Autodesk Inventor part; units mm, degrees
ref_plane "YZ Plane" through (0, 0, 0) normal (1, 0, 0) x (0, 1, 0)
ref_plane "XZ Plane" through (0, 0, 0) normal (0, 1, 0) x (-1, 0, 0)
ref_plane "XY Plane" through (0, 0, 0) normal (0, 0, 1) x (1, 0, 0)
sketch "Sketch1" plane through (0, 0, 0) normal (0, 1, 0) x (-1, 0, 0)
  line L0 (-20, 35) -> (20, 35)
  line L1 (20, 35) -> (20, -35)
  line L2 (20, -35) -> (-20, -35)
  line L3 (-20, -35) -> (-20, 35)
  line L4 (-20, 35) -> (20, -35) construction
  line L5 (20, 35) -> (-20, -35) construction
  circle A0 centre (0, 20) radius 2
  circle A1 centre (0, -20) radius 2
  line L6 (-12.5, 25) -> (12.5, 25) construction
  line L7 (12.5, 25) -> (12.5, -25) construction
  line L8 (12.5, -25) -> (-12.5, -25) construction
  line L9 (-12.5, -25) -> (-12.5, 25) construction
  line L10 (-12.5, 25) -> (12.5, -25) construction
  line L11 (12.5, 25) -> (-12.5, -25) construction
  circle A2 centre (12.5, -25) radius 5 construction
  circle A3 centre (12.5, -25) radius 1.5
  circle A4 centre (12.5, 25) radius 1.5
  circle A5 centre (-12.5, 25) radius 1.5
  circle A6 centre (-12.5, -25) radius 1.5
  point P0 (0, 0)
  dimension "d0" = 4
  dimension "d1" = 4
  dimension "d2" = 40
  dimension "d3" = 20
  dimension "d4" = 70
  dimension "d5" = 40
  dimension "d6" = 25
  dimension "d7" = 50
  dimension "d8" = 10
  dimension "d9" = 3
  dimension "d10" = 3
  dimension "d11" = 3
  dimension "d12" = 3
extrude "Extrusion1" add sketch "Sketch1" along normal blind 5
fillet "Fillet1" radius 2 4 edges at (20, 2.5, 35) (20, 2.5, -35) (-20, 2.5, -35) (-20, 2.5, 35)
chamfer "Chamfer1" distance 1.5 angle 45 4 edges at (-11, 5, 25) (14, 5, 25) (-11, 5, -25) (14, 5, -25)
properties part number "Encoder base"
Here's how the part is built. I have some questions about the finished solid (model axes, mm). Coordinates: 2 decimals unless noted, no trailing zeros. Order: outer loops, then holes, each group sorted by start corner. A loop starts at its lowest first (then second) coordinate and runs counter-clockwise, first axis right, second up. Notation, with made-up numbers: (48, 12.5) -> (79, 12.5) arc R28 cw to (79, 30.5) -> close; hole circle Ø6 at (48.25, -36). An arc over 180 degrees is marked (long way). Return JSON: item names as keys, results as strings.
1) If we section it at B-B on z = -20: List the corners of the cut face in (x, y) for me.
Conclusion:
{"outline": "(-20, 0) -> (-2, 0) -> (-2, 5) -> (-20, 5) -> close; (2, 0) -> (20, 0) -> (20, 5) -> (2, 5) -> close"}
2) If we section it at A-A on x = 0: List the corners of the cut face in (y, z) for me, plus the area to 3 significant figures.
Conclusion:
{"outline": "(0, -35) -> (5, -35) -> (5, -22) -> (0, -22) -> close; (0, -18) -> (5, -18) -> (5, 18) -> (0, 18) -> close; (0, 22) -> (5, 22) -> (5, 35) -> (0, 35) -> close", "area": "310 mm²"}
3) If we section it at D-D on x = 12.5: List the corners of the cut face in (y, z) for me.
Conclusion:
{"outline": "(0, -35) -> (5, -35) -> (5, -28) -> (3.5, -26.5) -> (0, -26.5) -> close; (0, -23.5) -> (3.5, -23.5) -> (5, -22) -> (5, 22) -> (3.5, 23.5) -> (0, 23.5) -> close; (0, 26.5) -> (3.5, 26.5) -> (5, 28) -> (5, 35) -> (0, 35) -> close"}
4) I'm going to push a flat-ended pin straight in: P1, Ø1.8, axis at x = 12.5, z = -25, coming from the +Y side. Where does the tip first touch, or does it pass through?
Conclusion:
{"P1": "passes through"}
5) Thinking about a two-plate mould opening in X: for faces 1 (the cylindrical face through (19.43, 2.54, -34.4)), 2 (the cylindrical face through (-12.305, 1.726, -26.487)), 3 (the cylindrical face through (-19.43, 2.54, 34.4)), which applies, +X half, -X half, draft (parallel to the pull), parting line (faces both ways), or undercut?
Conclusion:
{"face 1": "+X half", "face 2": "undercut", "face 3": "-X half"}
6) If I drill on probe 1 along Z at (x, y) = (-12.5, 2.7); probe 2 along X at (y, z) = (2.35, 26); probe 3 along Z at (x, y) = (1.5, 4.8), over which ranges is the centre line in solid material (lowest first)?
Conclusion:
{"probe 1": "z = -35 to -26.5, -23.5 to 23.5, 26.5 to 35", "probe 2": "x = -20 to -13.62, -11.38 to 11.38, 13.62 to 20", "probe 3": "z = -35 to -21.32, -18.68 to 18.68, 21.32 to 35"}
7) If we section it at C-C on y = 2.55: List the corners of the cut face in (x, z) for me, plus the area to 3 significant figures.
Conclusion:
{"outline": "(-20, -33) arc R2 ccw to (-18, -35) -> (18, -35) arc R2 ccw to (20, -33) -> (20, 33) arc R2 ccw to (18, 35) -> (-18, 35) arc R2 ccw to (-20, 33) -> close; hole circle Ø3 at (-12.5, -25); hole circle Ø3 at (-12.5, 25); hole circle Ø4 at (0, -20); hole circle Ø4 at (0, 20); hole circle Ø3 at (12.5, -25); hole circle Ø3 at (12.5, 25)", "area": "2,740 mm²"}
